Here's how the part is built. I have some questions about the finished solid (model axes, mm). A direction names the side the tool comes from. Round coordinates to 2 decimals unless told otherwise and drop trailing zeros. Write each loop counter-clockwise with the first axis right and the second up, starting at its lowest first coordinate (ties: lowest second). Pieces come first, ordered by that corner, then holes. Notation, with made-up numbers: (29.5, 51.5) -> (37.5, 51.5) arc R11 cw to (37.5, 65.5) -> close; hole circle Ø5 at (10.5, 40.25). An arc over 180 degrees is marked (long way). Put each result on its own line as item: value. Start each with the question number.
1. Suppose I cut it at C-C (y = -346.5). Please give me the cut outline in (x, z), then the cut area to 3 significant figures.
2. I need wall thicknesses on probe 1 along Z at (x, y) = (36, -180.5); probe 2 along Z at (x, y) = (57, -227). Which ranges of each line are inside material? Lowest first, please. Write a range as from..to.
3. For pin 1 (8 mm diameter, centred on x = 8.5, z = -42.5, fed in from +Y); pin 2 (1.5 mm diameter, centred on x = 23, y = -128.5, fed in from -Z); pin 3 (2 mm diameter, centred on x = 34.5, y = -115.5, fed in from -Z), each with a flat end and sliding along its axis, tell me the tip position at first contact or that it passes through.
4. Which directions (+Z, -Z, +X, -X, +Y, -Y) give clear straight access to the entire face, cutting with the end or side of a thin tool? Please do faces 4 (the face through (31.306, 31.154, -19.277)), 5 (the face through (31, -126, 0)).
5. We'd pull the mould along Y, two halves only. Please class faces 1 (the face through (31.306, -337.582, -28.514)), 2 (the face through (32.19, -260.2, 5.88)), 3 (the face through (63.5, -204, -79)): +Y half, -Y half, draft (parallel to the pull), parting line (faces both ways), or undercut.
6. Suppose I cut it at B-B (z = -72.5). Please give me the cut outline in (x, y), then the cut area to 3 significant figures.
7. Suppose I cut it at A-A (x = 29). Please give me the cut outline in (y, z).
```python
from build123d import *

# Parameters (mm, degrees)
F0_W      = 63.5
F0_H      = 6.35
F1_DEPTH  = 254.762
F2_W      = 63.5
F2_H      = 6.35
F3_ANGLE  = 20
F4_W      = 63.5
F4_H      = 6.35
F5_DEPTH  = 160.02
F6_W      = 63.5
F6_H      = 6.35
F7_ANGLE  = 160
F8_W      = 63.5
F8_H      = 6.35
F9_ANGLE  = 160
F11_DEPTH = 63.5


with BuildPart() as f1:
    # F0 (on Front) → F1 (new body)
    with BuildSketch(Plane.XZ):
        with Locations((31.75, 3.175)):
            Rectangle(F0_W, F0_H)
    extrude(amount=F1_DEPTH)

    # F2 (on face) → F3 (revolve)
    with BuildSketch(Plane.XZ.offset(254.762)):
        with Locations((31.75, 3.175)):
            Rectangle(F2_W, F2_H)
    revolve(axis=Axis((31.75, -254.762, -25.4), (1, 0, 0)), revolution_arc=F3_ANGLE)

    # F4 (on face) → F5 (join)
    with BuildSketch(Plane(origin=(0, -233.123909852, -84.8501640819), x_dir=(1, 0, 0), z_dir=(0, -0.9396926208, -0.3420201433))):
        with Locations((31.75, 91.840543186)):
            Rectangle(F4_W, F4_H)
    extrude(amount=F5_DEPTH)

    # F6 (on face) → F7 (revolve)
    with BuildSketch(Plane(origin=(0, -383.4935230301, -139.5802274168), x_dir=(1, 0, 0), z_dir=(0, -0.9396926208, -0.3420201433))):
        with Locations((31.75, 91.840543186)):
            Rectangle(F6_W, F6_H)
    revolve(axis=Axis((31.75, -405.1316131782, -80.130063335), (1, 0, 0)), revolution_arc=F7_ANGLE)

    # F8 (on face) → F9 (revolve)
    with BuildSketch(Plane(origin=(0, 0, 0), x_dir=(-1, 0, 0), z_dir=(0, 1, 0))):
        with Locations((-31.75, 3.175)):
            Rectangle(F8_W, F8_H)
    revolve(axis=Axis((31.75, 0, -25.4), (-1, 0, 0)), revolution_arc=F9_ANGLE)

    # F10 (on face) → F11 (join)
    with BuildSketch(Plane.YZ.offset(63.5)):
        Polygon((-405.1316131782, -105.530063335), (-405.1316131782, -111.880063335), (10.8591395506, -55.23524071), (8.6873116405, -49.268192568), align=None)
    extrude(amount=-F11_DEPTH)


solid = f1.part
```
Verdict:
1. outline: (0, -103.9) -> (63.5, -103.9) -> (63.5, -97.56) -> (0, -97.56) -> close; (0, -31.76) -> (63.5, -31.76) -> (63.5, -25) -> (0, -25) -> close
1. area: 832 mm^2
2. probe 1: z = -81.29..-74.99, 0..6.35
2. probe 2: z = -87.62..-81.31, 0..6.35
3. pin 1: stops at y = 28.92
3. pin 2: stops at z = -74.31
3. pin 3: stops at z = -72.58
4. face 4: +X, -X, +Y
4. face 5: +X, -X
5. face 1: undercut
5. face 2: -Y half
5. face 3: draft
6. outline: (0, -435.95) -> (63.5, -435.95) -> (63.5, -429.36) -> (0, -429.36) -> close; (0, -162.19) -> (63.5, -162.19) -> (63.5, -115.93) -> (0, -115.93) -> close
6. area: 3,360 mm^2
7. outline: (-415.99, -50.29) arc R31.75 ccw to (-405.13, -111.88) -> (10.86, -55.24) arc R31.75 ccw to (0, 6.35) -> (-254.76, 6.35) arc R31.75 ccw to (-265.62, 4.44) -> close; hole (-413.82, -56.26) arc R25.4 ccw to (-405.13, -105.53) -> (8.69, -49.27) arc R25.4 ccw to (0, 0) -> (-254.76, 0) arc R25.4 ccw to (-263.45, -1.53) -> close
